Autodesk Inventor part; units mm, degrees
ref_plane "YZ Plane" through (0, 0, 0) normal (1, 0, 0) x (0, 1, 0)
ref_plane "XZ Plane" through (0, 0, 0) normal (0, 1, 0) x (-1, 0, 0)
ref_plane "XY Plane" through (0, 0, 0) normal (0, 0, 1) x (1, 0, 0)
sketch "Sketch1" plane through (0, 0, 0) normal (0, 0, 1) x (1, 0, 0)
  line L0 (-150, 150) -> (150, 150)
  line L1 (150, 150) -> (150, -150)
  line L2 (150, -150) -> (-150, -150)
  line L3 (-150, -150) -> (-150, 150)
  point P0 (0, 0)
  point P1 (150, 0)
  point P2 (0, 150)
  dimension "d0" = 300
  dimension "d1" = 300
extrude "Extrusion1" add sketch "Sketch1" along normal blind 10
sketch "Sketch2" plane through (0, 0, 10) normal (0, 0, 1) x (1, 0, 0)
  line L0 (-150, 150) -> (150, 150)
  line L1 (150, 150) -> (150, -150)
  line L2 (150, -150) -> (-150, -150)
  line L3 (-150, -150) -> (-150, 150)
  line L4 (140, 140) -> (-140, 140)
  line L5 (-140, 140) -> (-140, -140)
  line L6 (-140, -140) -> (140, -140)
  line L7 (140, -140) -> (140, 140)
  point P0 (0, 0)
  dimension "d4" = 10
extrude "Extrusion2" add sketch "Sketch2" along normal blind 100
sketch "Sketch3" plane through (-150, -150, 0) normal (-1, 0, 0) x (0, 0, 1)
  circle A0 centre (60, 250) radius 12.5
  circle A1 centre (90, 50) radius 13.3073
  line L0 (0, 300) -> (110, 300)
  line L1 (0, 0) -> (110, 0)
  line L2 (110, 300) -> (110, 0)
  point P0 (0, 150)
  dimension "d7" = 25
  dimension "d8" = 50
  dimension "d9" = 50
  dimension "d10" = 20
  dimension "d11" = 50
sketch "Sketch6" plane through (0, 0, 0) normal (0, 0, -1) x (-1, 0, 0)
  circle A0 centre (0, 0) radius 59.25
  dimension "d21" = 118.5
extrude "Extrusion6" cut sketch "Sketch6" against normal blind 5
sketch "Sketch7" plane through (0, 0, 5) normal (0, 0, -1) x (-1, 0, 0)
  circle A0 centre (42.997, -32.6689) radius 2
  line L0 (42.997, -32.6689) -> (0, 0) construction
  dimension "d24" = 54
  dimension "d25" = 4
extrude "Extrusion7" cut sketch "Sketch7" against normal up to surface (5 mm away)
pattern_circular "Circular Pattern1" count 10 over 360 about axis through (0, 0, 5) along (0, 0, 1) of "Extrusion7"
extrude "Extrusion8" cut sketch "Sketch3" against normal blind 10 contours A1
sketch "Sketch8" plane through (-150, -150, 0) normal (-1, 0, 0) x (0, 0, 1)
  circle A0 centre (90, 75.4) radius 2.05
  circle A1 centre (90, 24.6) radius 2.05
  line L0 (90, 24.6) -> (90, 75.4) construction
  line L1 (0, 0) -> (0, 300) construction
  circle A2 centre (90, 50) radius 13.3073 construction
  circle A3 centre (90, 50) radius 13.3073 construction
  point P0 (0, 150)
  dimension "d33" = 4.1
  dimension "d34" = 4.1
  dimension "d35" = 50.8
  dimension "d37" = 0
extrude "Extrusion9" cut sketch "Sketch8" against normal blind 10
sketch "Sketch9" plane through (0, 0, 110) normal (0, 0, 1) x (1, 0, 0)
  circle A0 centre (-145, -145) radius 2.05
  circle A1 centre (-145, 145) radius 2.05
  line L0 (-145, -145) -> (-145, 145) construction
  line L1 (-150, 150) -> (-150, -150) construction
  line L2 (-150, -150) -> (150, -150) construction
  point P0 (0, 0)
  point P1 (-145, 0)
  point P2 (-150, 0)
  dimension "d40" = 4.1
  dimension "d41" = 4.1
  dimension "d42" = 5
  dimension "d44" = 5
extrude "Extrusion10" cut sketch "Sketch9" against normal blind 10
mirror "Mirror2" about plane through (0, 0, 0) normal (1, 0, 0) of "Extrusion8", "Extrusion9", "Extrusion10"
properties part number "locomotion box"
Build history of the part. All positions in model axes, mm. A direction names the side the tool comes from. Give positions to 0.01 mm unless a question says otherwise; leave off trailing zeros. Loops run counter-clockwise (first coordinate to the right, second up) from the corner with the lowest first, then second, coordinate; pieces in that order, holes last.
1) Band-saw the part on A-A on z = 14.5. List the corners of the cut face in (x, y).
Values follow:
outline: (-150, -150) - (150, -150) - (150, 150) - (-150, 150) - close; hole (-140, -140) - (140, -140) - (140, 140) - (-140, 140) - close
2) Band-saw the part on B-B on y = 105. List the corners of the cut face in (x, z).
Values follow:
outline: (-150, 0) - (150, 0) - (150, 110) - (140, 110) - (140, 10) - (-140, 10) - (-140, 110) - (-150, 110) - close
3) Drop flat-ended pins along their axis: P1, Ø3.5, axis at x = -146, y = -144.5, coming from the +Z side; P2, Ø2, axis at x = 120, y = -24, coming from the +Z side. Give the stop position or say it passes through.
Values follow:
P1: stops at z = 110
P2: stops at z = 10
4) 3-axis set-ups, long thin cutter, end or side, ignore diameter. For faces 4 (the face through (2, 140, 59)), 5 (the face through (145.07, -91.9, 79.44)), 6 (the face through (59.193, 2.605, 2.465)): which of +Z, -Z, +X, -X, +Y, -Y reach the whole face in a straight line?
Values follow:
face 4: +Z
face 5: +X, -X
face 6: -Z
5) Probe line 1 along Y through (x, z) = (21.5, 22); line 2 along Z through (x, y) = (-62.5, -58). List the from-to ranges inside material, lowest first.
Values follow:
line 1: y = -150 to -140, 140 to 150
line 2: z = 0 to 10
6) Band-saw the part on C-C on x = 0. List the corners of the cut face in (y, z), then the cut area to 3 significant figures.
Values follow:
outline: (-150, 0) - (-59.25, 0) - (-59.25, 5) - (59.25, 5) - (59.25, 0) - (150, 0) - (150, 110) - (140, 110) - (140, 10) - (-140, 10) - (-140, 110) - (-150, 110) - close
area: 4,410 mm2
7) Two-plate mould, pull along Y, no slides. Class faces 1 (the face through (-150, -2, 54)), 2 (the face through (2, -150, 54)), 3 (the face through (-2, 2, 10)): released by +Y, released by -Y, zero draft, split by the parting line, or undercut.
Values follow:
face 1: zero draft
face 2: released by -Y
face 3: undercut
8) Band-saw the part on D-D on y = 7.5. List the corners of the cut face in (x, z).
Values follow:
outline: (-150, 0) - (-58.77, 0) - (-58.77, 5) - (58.77, 5) - (58.77, 0) - (150, 0) - (150, 110) - (140, 110) - (140, 10) - (-140, 10) - (-140, 110) - (-150, 110) - close
